```python
from build123d import *

# Parameters (mm, degrees)
SKETCH_1_R        = 2.8
EXTRUDE_1_DEPTH   = 8
EXTRUDE_1_2_DEPTH = 8
EXTRUDE_1_3_DEPTH = 8
SKETCH_2_W        = 51.3875
SKETCH_2_H        = 18.05
EXTRUDE_2_DEPTH   = 1
SKETCH_3_W        = 51.3875
SKETCH_3_H        = 18.05
SKETCH_3_W_2      = 49.3875
SKETCH_3_H_2      = 16.05
EXTRUDE_3_DEPTH   = 9
SKETCH_4_W        = 7.50625
SKETCH_4_H        = 1.2
SKETCH_4_W_2      = 1.2
SKETCH_4_H_2      = 5.825
SKETCH_4_W_3      = 10.5875
EXTRUDE_4_DEPTH   = 2.5
FILLET_1_R        = 5
FILLET_2_R        = 1.6


with BuildPart() as part:
    # Sketch 1 → Extrude 1 (new body)
    with BuildSketch(Plane(origin=(0, 0, 0), x_dir=(1, 0, 0), z_dir=(0, 1, 0))):
        with Locations(Location((0, 0, 0), (0, 0, 270))):
            Circle(SKETCH_1_R)
        Polygon((2.2, 0.6), (2.2, -0.6), (0.6, -0.6), (0.6, -2.2), (-0.6, -2.2), (-0.6, -0.6), (-2.2, -0.6), (-2.2, 0.6), (-0.6, 0.6), (-0.6, 2.2), (0.6, 2.2), (0.6, 0.6), align=None, mode=Mode.SUBTRACT)
    extrude(amount=-EXTRUDE_1_DEPTH)

    # Sketch 2 → Extrude 2 (add)
    with BuildSketch(Plane(origin=(0, 0, 0), x_dir=(1, 0, 0), z_dir=(0, 1, 0))):
        Rectangle(SKETCH_2_W, SKETCH_2_H)
    extrude(amount=EXTRUDE_2_DEPTH)

    # Sketch 3 → Extrude 3 (add)
    with BuildSketch(Plane(origin=(0, 0, 0), x_dir=(1, 0, 0), z_dir=(0, 1, 0))):
        Rectangle(SKETCH_3_W, SKETCH_3_H)
        Rectangle(SKETCH_3_W_2, SKETCH_3_H_2, mode=Mode.SUBTRACT)
    extrude(amount=-EXTRUDE_3_DEPTH)



with BuildPart() as body_2:
    # Sketch 1 → Extrude 1 2 (new body)
    with BuildSketch(Plane(origin=(0, 0, 0), x_dir=(1, 0, 0), z_dir=(0, 1, 0))):
        with Locations(Location((-11.90625, 0, 0), (0, 0, 270))):
            Circle(SKETCH_1_R)
        Polygon((-14.10625, -0.6), (-14.10625, 0.6), (-12.50625, 0.6), (-12.50625, 2.2), (-11.30625, 2.2), (-11.30625, 0.6), (-9.70625, 0.6), (-9.70625, -0.6), (-11.30625, -0.6), (-11.30625, -2.2), (-12.50625, -2.2), (-12.50625, -0.6), align=None, mode=Mode.SUBTRACT)
    extrude(amount=-EXTRUDE_1_2_DEPTH)


with BuildPart() as body_3:
    # Sketch 1 → Extrude 1 3 (new body)
    with BuildSketch(Plane(origin=(0, 0, 0), x_dir=(1, 0, 0), z_dir=(0, 1, 0))):
        with Locations(Location((11.90625, 0, 0), (0, 0, 270))):
            Circle(SKETCH_1_R)
        Polygon((9.70625, 0.6), (9.70625, -0.6), (11.30625, -0.6), (11.30625, -2.2), (12.50625, -2.2), (12.50625, -0.6), (14.10625, -0.6), (14.10625, 0.6), (12.50625, 0.6), (12.50625, 2.2), (11.30625, 2.2), (11.30625, 0.6), align=None, mode=Mode.SUBTRACT)
    extrude(amount=-EXTRUDE_1_3_DEPTH)


with BuildPart() as part_1:
    add(part.part)

    add(body_2.part)  # Extrude 4 merges body 2

    add(body_3.part)  # Extrude 4 merges body 3
    # Sketch 4 → Extrude 4 (add)
    with BuildSketch(Plane(origin=(0, 0, 0), x_dir=(1, 0, 0), z_dir=(0, 1, 0))):
        with Locations((5.953125, 0)):
            Rectangle(SKETCH_4_W, SKETCH_4_H)
        with Locations((11.90625, 5.1125)):
            Rectangle(SKETCH_4_W_2, SKETCH_4_H_2)
        with Locations((11.90625, -5.1125)):
            Rectangle(SKETCH_4_W_2, SKETCH_4_H_2)
        with Locations((19.4, 0)):
            Rectangle(SKETCH_4_W_3, SKETCH_4_H)
        with Locations((0, 5.1125)):
            Rectangle(SKETCH_4_W_2, SKETCH_4_H_2)
        with Locations((-5.953125, 0)):
            Rectangle(SKETCH_4_W, SKETCH_4_H)
        with Locations((0, -5.1125)):
            Rectangle(SKETCH_4_W_2, SKETCH_4_H_2)
        with Locations((-11.90625, 5.1125)):
            Rectangle(SKETCH_4_W_2, SKETCH_4_H_2)
        with Locations((-11.90625, -5.1125)):
            Rectangle(SKETCH_4_W_2, SKETCH_4_H_2)
        with Locations((-19.4, 0)):
            Rectangle(SKETCH_4_W_3, SKETCH_4_H)
    extrude(amount=-EXTRUDE_4_DEPTH)

    # Fillet 1
    fillet_1_edges = [part_1.edges().sort_by_distance(p)[0] for p in [
        (25.69375, -4, 9.025),
        (25.69375, -4, -9.025),
        (-25.69375, -4, -9.025),
        (-25.69375, -4, 9.025),
        (-24.69375, -4.5, 8.025),
        (-24.69375, -4.5, -8.025),
        (24.69375, -4.5, -8.025),
        (24.69375, -4.5, 8.025),
    ]]
    fillet(fillet_1_edges, radius=FILLET_1_R)

    # Fillet 2
    fillet_2_edges = [part_1.edges().sort_by_distance(p)[0] for p in [
        (5.953125, 0, -8.025),
        (16.1, 0, 8.025),
        (24.69375, 0, -1.8125),
        (-5.953125, 0, -8.025),
        (5.953125, 0, 8.025),
        (-16.1, 0, -8.025),
        (-5.953125, 0, 8.025),
        (-24.69375, 0, 1.8125),
        (-25.69375, 1, 0),
        (0, 1, -9.025),
        (25.69375, 1, 0),
        (0, 1, 9.025),
        (-24.229283906, 1, 7.560533906),
        (24.229283906, 1, 7.560533906),
        (24.229283906, 1, -7.560533906),
        (-24.229283906, 1, -7.560533906),
        (-24.69375, 0, -1.8125),
        (-23.229283906, 0, -6.560533906),
        (16.1, 0, -8.025),
        (23.229283906, 0, -6.560533906),
        (24.69375, 0, 1.8125),
        (23.229283906, 0, 6.560533906),
        (-16.1, 0, 8.025),
        (-23.229283906, 0, 6.560533906),
    ]]
    fillet(fillet_2_edges, radius=FILLET_2_R)


solid = part_1.part
```
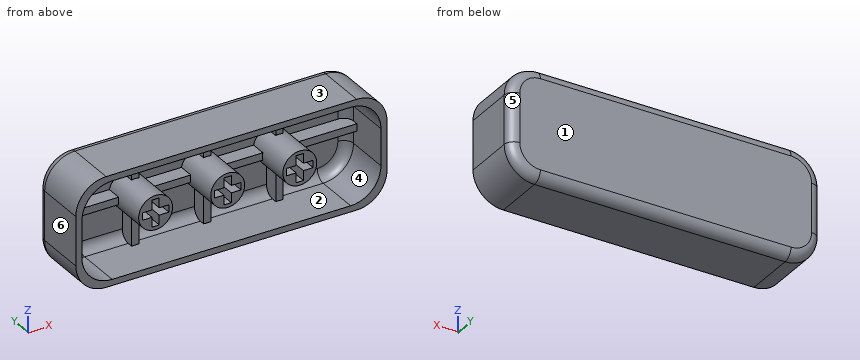
Build history of the part. All positions in model axes, mm. Face numbers are marked on the shaded views. A direction names the side the tool comes from. Round coordinates to 2 decimals unless told otherwise and drop trailing zeros. Order: outer loops, then holes, each group sorted by start corner. A loop starts at its lowest first (then second) coordinate and runs counter-clockwise, first axis right, second up. Notation, with made-up numbers: (87.5, 75) -> (139.5, 75) arc R20 cw to (139.5, 99) -> close; hole circle Ø9 at (49, 76). An arc over 180 degrees is marked (long way). Answer in a Markdown table with one row per item.
1) Which spindle directions (+Z, -Z, +X, -X, +Y, -Y) get a long thin tool onto all of the face, cutting with end or side? Do the marked faces 1 and 2. Say none if no direction does.
Values:
| item | result |
|---|---|
| face 1 | +Z, -Z, +X, -X, +Y |
| face 2 | -Y |
2) Mould opens along X. For the marked faces 3, 4, 5 and 6 say: released by +X, released by -X, zero draft, split by the parting line, or undercut.
Values:
| item | result |
|---|---|
| face 3 | zero draft |
| face 4 | undercut |
| face 5 | released by +X |
| face 6 | released by -X |
3) Band-saw the part on D-D on y = -5. Give the number of separate pieces and of enclosed holes in the cut face, and give its area (3 significant figures).
Values:
| item | result |
|---|---|
| separate pieces | 4 |
| enclosed holes | 4 |
| area | 181 mm2 |
4) Band-saw the part on B-B on x = -8. Give the cut face in (y, z) (3 decimals), and give its area (4 significant figures).
Values:
| item | result |
|---|---|
| outline | (-9, -9.025) -> (-0.6, -9.025) arc R1.6 ccw to (1, -7.425) -> (1, 7.425) arc R1.6 ccw to (-0.6, 9.025) -> (-9, 9.025) -> (-9, 8.025) -> (-1.6, 8.025) arc R1.6 cw to (0, 6.425) -> (0, 0.6) -> (-2.5, 0.6) -> (-2.5, -0.6) -> (0, -0.6) -> (0, -6.425) arc R1.6 cw to (-1.6, -8.025) -> (-9, -8.025) -> close |
| area | 39.05 mm2 |
5) Pin check, flat tips, straight feed: P1, Ø1.3, axis at x = 0, z = -4, coming from the -Y side; P2, Ø6.5, axis at x = -7.5, z = -3.5, coming from the -Y side; P3, Ø1.2, axis at y = -1, z = 6, coming from the +X side. Stop position of each tip, or through.
Values:
| item | result |
|---|---|
| P1 | y = -2.5 |
| P2 | y = -8 |
| P3 | x = 25.5 |
6) Wall check: L1, parallel to Z at x = 6, y = -1.75 (3 decimals); L2, parallel to Z at x = 6.5, y = -7.75 (3 decimals); L3, parallel to Z at x = 2, y = -7.5 (3 decimals). Give the ranges that are in metal, low to high.
Values:
| item | result |
|---|---|
| L1 | -9.025 to -8.025, -0.6 to 0.6, 8.025 to 9.025 |
| L2 | -9.025 to -8.025, 8.025 to 9.025 |
| L3 | -9.025 to -8.025, -1.96 to -0.6, 0.6 to 1.96, 8.025 to 9.025 |
7) Band-saw the part on C-C on y = 0.5. Give the cut face in (x, z) (3 decimals).
Values:
| item | result |
|---|---|
| outline | (-25.256, -4.025) arc R4.562 ccw to (-20.694, -8.587) -> (20.694, -8.587) arc R4.562 ccw to (25.256, -4.025) -> (25.256, 4.025) arc R4.562 ccw to (20.694, 8.587) -> (-20.694, 8.587) arc R4.562 ccw to (-25.256, 4.025) -> close |
